```python
from build123d import *

# Parameters (mm, degrees)
F0_W      = 60
F0_H      = 30
F1_DEPTH  = 60
F2_R      = 3.4
F3_DEPTH  = 60.001
F4_R      = 1.8
F5_DEPTH  = 30.001
F7_DEPTH  = 7
F9_DEPTH  = 7
F11_DEPTH = 7
F13_DEPTH = 7
F14_R     = 17.5
F15_DEPTH = 12
F17_DEPTH = 30.001
F18_SIZE  = 2


with BuildPart() as f1:
    # F0 (on Top) → F1 (new body)
    with BuildSketch(Plane.XY):
        Rectangle(F0_W, F0_H)
    extrude(amount=F1_DEPTH)

    # F2 (on face) → F3 (cut, through all)
    with BuildSketch(Plane.XY.offset(60)):
        with Locations((0, 15)):
            Circle(F2_R)
    extrude(amount=-F3_DEPTH, mode=Mode.SUBTRACT)

    # F4 (on face) → F5 (cut, through all)
    with BuildSketch(Plane.XZ.offset(15)):
        with Locations((-23, 53)):
            Circle(F4_R)
        with Locations((23, 53)):
            Circle(F4_R)
        with Locations((23, 7)):
            Circle(F4_R)
        with Locations((-23, 7)):
            Circle(F4_R)
    extrude(amount=-F5_DEPTH, mode=Mode.SUBTRACT)

    # F6 (on face) → F7 (cut)
    with BuildSketch(Plane.XZ.offset(15)):
        Polygon((-23, 48.3811978465), (-19, 50.6905989232), (-19, 55.3094010768), (-23, 57.6188021535), (-27, 55.3094010768), (-27, 50.6905989232), align=None)
    extrude(amount=-F7_DEPTH, mode=Mode.SUBTRACT)

    # F8 (on face) → F9 (cut)
    with BuildSketch(Plane.XZ.offset(15)):
        Polygon((19, 50.6905989232), (23, 48.3811978465), (27, 50.6905989232), (27, 55.3094010768), (23, 57.6188021535), (19, 55.3094010768), align=None)
    extrude(amount=-F9_DEPTH, mode=Mode.SUBTRACT)

    # F10 (on face) → F11 (cut)
    with BuildSketch(Plane.XZ.offset(15)):
        Polygon((-23, 2.3811978465), (-19, 4.6905989232), (-19, 9.3094010768), (-23, 11.6188021535), (-27, 9.3094010768), (-27, 4.6905989232), align=None)
    extrude(amount=-F11_DEPTH, mode=Mode.SUBTRACT)

    # F12 (on face) → F13 (cut)
    with BuildSketch(Plane.XZ.offset(15)):
        Polygon((23, 2.3811978465), (27, 4.6905989232), (27, 9.3094010768), (23, 11.6188021535), (19, 9.3094010768), (19, 4.6905989232), align=None)
    extrude(amount=-F13_DEPTH, mode=Mode.SUBTRACT)

    # F14 (on face) → F15 (join)
    with BuildSketch(Plane.XZ.offset(15)):
        with Locations((0, 60)):
            Circle(F14_R)
    extrude(amount=-F15_DEPTH)

    # F16 (on face) → F17 (cut, through all)
    with BuildSketch(Plane.XZ.offset(15)):
        with BuildLine():
            Line((-12.5, 60), (12.5, 60))
            ThreePointArc((12.5, 60), (0, 72.5), (-12.5, 60))
        make_face()
    extrude(amount=-F17_DEPTH, mode=Mode.SUBTRACT)

    # F18
    f18_edges = [f1.edges().sort_by_distance(p)[0] for p in [
        (0, -15, 77.5),
        (0, -3, 77.5),
        (0, -15, 72.5),
        (0, -3, 72.5),
    ]]
    chamfer(f18_edges, length=F18_SIZE)


solid = f1.part
```
Work out the finished part from the listing and answer in its coordinate system (mm). A direction names the side the tool comes from. Give positions to 0.01 mm unless a question says otherwise; leave off trailing zeros. Loops run counter-clockwise (first coordinate to the right, second up) from the corner with the lowest first, then second, coordinate; pieces in that order, holes last. Notation, with made-up numbers: (7.5, 46.5) - (58.5, 46.5) arc R32 cw to (58.5, 85.5) - close; hole circle Ø5 at (40, -33.75). An arc over 180 degrees is marked (long way). One line per question, with ' | ' between items.
(1) The part is cut by section C-C (x = 0). Write down the section's boundary in (y, z), then the cut area to 3 significant figures.
Recorded:
outline: (-15, 0) - (11.6, 0) - (11.6, 60) - (-15, 60) - close; (-15, 74.5) - (-13, 72.5) - (-5, 72.5) - (-3, 74.5) - (-3, 75.5) - (-5, 77.5) - (-13, 77.5) - (-15, 75.5) - close | area: 1,650 mm²
(2) The part is cut by section B-B (y = 0). Write down the section's boundary in (x, z).
Recorded:
outline: (-30, 0) - (30, 0) - (30, 60) - (-30, 60) - close; hole circle Ø3.6 at (-23, 7); hole circle Ø3.6 at (-23, 53); hole circle Ø3.6 at (23, 7); hole circle Ø3.6 at (23, 53)
(3) A tool of negligible diameter and unlimited length cuts with its end or side. For faces 3 (the face through (30, 0, 30)), 4 (the face through (0.275, -9.056, 72.497)), 5 (the face through (-24.97, -11.55, 10.48)), from which of +Z, -Z, +X, -X, +Y, -Y can it reach the whole face along a straight path? Write none if from no direction.
Recorded:
face 3: +Z, -Z, +X, +Y, -Y | face 4: +Y, -Y | face 5: -Y
(4) Each of these flat-tipped pins is pushed along its axis until it touches: pin 1 Ø9 at (x, y) = (2.5, -5.5) entering from +Z; pin 2 Ø5 at (x, y) = (13.5, -5) entering from +Z; pin 3 Ø4 at (x, z) = (-24.5, 54) entering from -Y; pin 4 Ø8 at (y, z) = (-1.5, 69) entering from -X. Where does it stop, or does it pass through?
Recorded:
pin 1: stops at z = 77.5 | pin 2: stops at z = 73.61 | pin 3: stops at y = -8 | pin 4: stops at x = -16.01
(5) The mould has two halves that part along Z. Classify faces 1 (the face through (0, -3, 75)), 2 (the face through (-27, -12, 53)): +Z half, -Z half, draft (parallel to the pull), parting line (faces both ways), or undercut.
Recorded:
face 1: draft | face 2: undercut
(6) Straight lines are drawn through the part: probe 1 along Z at (x, y) = (23, -0.25); probe 2 along Z at (x, y) = (19.5, -12.5); probe 3 along Z at (x, y) = (-13, 0.5). For each, find the intervals that lie inside material, in ascending order.
Recorded:
probe 1: z = 0 to 5.2, 8.8 to 51.2, 54.8 to 60 | probe 2: z = 0 to 4.4, 9.6 to 50.4, 55.6 to 60 | probe 3: z = 0 to 60
(7) The part is cut by section A-A (z = 53). Write down the section's boundary in (x, y), then the cut area to 3 significant figures.
Recorded:
outline: (-30, -15) - (-27, -15) - (-27, -8) - (-24.8, -8) - (-24.8, 15) - (-30, 15) - close; (-21.2, -8) - (-19, -8) - (-19, -15) - (19, -15) - (19, -8) - (21.2, -8) - (21.2, 15) - (3.4, 15) arc R3.4 cw to (-3.4, 15) - (-21.2, 15) - close; (24.8, -8) - (27, -8) - (27, -15) - (30, -15) - (30, 15) - (24.8, 15) - close | area: 1,500 mm²
